Autodesk Inventor part; units mm, degrees
ref_plane "Start Plane" through (0, 0, -85) normal (0, 0, 1) x (1, 0, 0)
ref_plane "End Plane" through (0, 0, 1585) normal (0, 0, 1) x (1, 0, 0)
ref_plane "Work Plane4" through (85, 0, 1585) normal (-0.7071, 0, 0.7071) x (0.7071, 0, 0.7071)
ref_plane "Start Plane" through (0, 0, -85) normal (0, 0, 1) x (1, 0, 0)
ref_plane "End Plane" through (0, 0, 1585) normal (0, 0, 1) x (1, 0, 0)
sketch "Sketch" plane through (0, 0, 0) normal (0, 0, 1) x (1, 0, 0)
  line L0 (-85, 167.3) -> (-22, 167.3)
  line L1 (-85, 180) -> (-85, 167.3)
  line L2 (85, 180) -> (-85, 180)
  line L3 (85, 167.3) -> (85, 180)
  line L4 (22, 167.3) -> (85, 167.3)
  line L5 (4, -149.3) -> (4, 149.3)
  line L6 (85, -167.3) -> (22, -167.3)
  line L7 (85, -180) -> (85, -167.3)
  line L8 (-85, -167.3) -> (-85, -180)
  line L9 (-22, -167.3) -> (-85, -167.3)
  line L10 (-4, 149.3) -> (-4, -149.3)
  line L11 (0, -252) -> (0, 252) construction
  line L12 (-4, -167.3) -> (4, -167.3) construction
  arc A0 (-22, -167.3) -> (-4, -149.3) centre (-22, -149.3) ccw
  arc A1 (-4, 149.3) -> (-22, 167.3) centre (-22, 149.3) ccw
  arc A2 (22, 167.3) -> (4, 149.3) centre (22, 149.3) ccw
  arc A3 (4, -149.3) -> (22, -167.3) centre (22, -149.3) ccw
  line L13 (-119, 0) -> (119, 0) construction
  line L14 (-85, -180) -> (85, -180)
  point P0 (-4, 167.3)
  point P1 (4, 167.3)
  point P2 (0, 0)
  point P3 (0, -167.3)
  point P4 (0, 0)
  dimension "d1" = 360
  dimension "d3" = 12.7
  dimension "d5" = 8
  dimension "d7" = 170
  dimension "d13" = 18
  dimension "d14" = 180
  dimension "d15" = 85
extrude "Body" add sketch "Sketch" along normal up to surface (1670 mm away) from surface at -85
sketch "Sketch3" plane through (0, 0, 0) normal (0, 0, 1) x (1, 0, 0)
  line L0 (0, 0) -> (10, 0)
ref_plane "Work Plane3" through (0, 0, 0) normal (0, -1, 0) x (1, 0, 0)
ref_plane "Work Plane4" through (85, 0, 1585) normal (-0.7071, 0, 0.7071) x (0.7071, 0, 0.7071)
split "Split1" plane through (85, 0, 1585) removes the side toward (-0.7071, 0, 0.7071)
ref_plane "Work Plane5" through (85, 0, -85) normal (-0.7071, 0, -0.7071) x (-0.7071, 0, 0.7071)
split "Split2" plane through (85, 0, -85) removes the side toward (-0.7071, 0, -0.7071)
sketch "Sketch4" plane through (0, 0, 0) normal (0, -1, 0) x (1, 0, 0)
  line L0 (-2, -85) -> (12, -85)
  line L1 (-2, 1585) -> (12, 1585)
  dimension "d19" = 1670
equation "\"d1\" = ParH"
equation "\"d3\" = t2"
equation "\"d7\" = b"
equation "\"d13\" = R1"
equation "\"d14\" = 0.5 * d1"
equation "\"d15\" = 0.5 * d7"
equation "\"d8\" = G_L"
equation "\"b\" = 170"
equation "\"ParH\" = 360"
equation "\"R1\" = 18"
equation "\"G_L\" = d19"
equation "\"t1\" = 8"
equation "\"t2\" = 12.7"
equation "\"G_OFFSET_START\" = 85"
equation "\"G_OFFSET_END\" = 85"
equation "\"d16\" = -G_OFFSET_START"
equation "\"d17\" = G_OFFSET_END + B_L"
properties part number "DIN 1025 - IPE 360-1670" material "Steel, Mild"
Design review of the part built by this model. Coordinates are the model's own, in mm. A direction names the side the tool comes from. Give positions to 0.01 mm unless a question says otherwise; leave off trailing zeros. Order: outer loops, then holes, each group sorted by start corner. A loop starts at its lowest first (then second) coordinate and runs counter-clockwise, first axis right, second up. Notation, with made-up numbers: M 50.5,17.5 L 102.5,17.5 A21 cw 102.5,41.5 Z; hole C -4,45 d10. An arc over 180 degrees is marked long. One line per question, with ' | ' between items. Start each with the question number.
Q1. We need section B-B (z = 1254). Write out the cut boundary in (x, y), plus the area to 3 significant figures.
Q2. For L1, parallel to Y at x = 34.5, z = 111; L2, parallel to X at y = -38.5, z = 1379; L3, parallel to Y at x = 17.5, z = 228, list the stretches that pass through material, from the lowest coordinate up. Write a range as [from, to].
Q3. Machinability: for faces 4 (the face through (-54, 167.3, 740)), 5 (the face through (4, -2, 739)), 6 (the face through (0, 1, 0)), which of the approach directions +Z, -Z, +X, -X, +Y, -Y give a long, thin tool a straight path to every point of the face, cutting with its end or side? Answer none if there is none.
Q4. The part is to be moulded in two halves that separate along Y. For faces 1 (the face through (0, -1, 1500)), 2 (the face through (53, 167.3, 738)), 3 (the face through (1, 180, 738)), say which applies: +Y half, -Y half, draft (parallel to the pull), parting line (faces both ways), or undercut.
Q5. We need section C-C (y = -19). Write out the cut boundary in (x, z), plus the area to 3 significant figures.
Q6. For pin 1 Ø1 at (y, z) = (52.5, 165) entering from +X; pin 2 Ø3 at (y, z) = (90, 965) entering from -X, all flat-tipped, find the tip position at first contact; note any pin that passes through.
Q7. We need section A-A (x = 41.5). Write out the cut boundary in (y, z), plus the area to 3 significant figures.
Returned:
1) outline: M -85,-180 L 85,-180 L 85,-167.3 L 22,-167.3 A18 cw 4,-149.3 L 4,149.3 A18 cw 22,167.3 L 85,167.3 L 85,180 L -85,180 L -85,167.3 L -22,167.3 A18 cw -4,149.3 L -4,-149.3 A18 cw -22,-167.3 L -85,-167.3 Z | area: 7,270 mm2
2) L1: [-180, -167.3], [167.3, 180] | L2: [-4, 4] | L3: [-180, -166.73], [166.73, 180]
3) face 4: +Z, -Z, -X | face 5: +Z, -Z, +X | face 6: -Z, -X, +Y, -Y
4) face 1: draft | face 2: undercut | face 3: +Y half
5) outline: M -4,4 L 4,-4 L 4,1504 L -4,1496 Z | area: 12,000 mm2
6) pin 1: x = 4 | pin 2: x = -4
7) outline: M -180,-41.5 L -167.3,-41.5 L -167.3,1541.5 L -180,1541.5 Z; M 167.3,-41.5 L 180,-41.5 L 180,1541.5 L 167.3,1541.5 Z | area: 40,200 mm2
